Can you work these out from the drawing? Everything is in mm from the part's minimum corner. Coordinates: 2 decimals unless noted, no trailing zeros. Write each loop counter-clockwise with the first axis right and the second up, starting at its lowest first coordinate (ties: lowest second). Pieces come first, ordered by that corner, then holes.
(1) Thinking about a two-plate mould opening in Y: for the marked faces 1, 2 and 3, which applies, released by +Y, released by -Y, zero draft, split by the parting line, or undercut?
(2) Imagine slicing it at A-A, the plane x = 22.5. List the corners of the cut face in (y, z) for me.
(3) Imagine slicing it at B-B, the plane y = 22.5. List the corners of the cut face in (x, z) for me, plus the area to 3 significant figures.
(4) Imagine slicing it at D-D, the plane x = 30.5. List the corners of the cut face in (y, z) for me, plus the area to 3 significant figures.
(5) Imagine slicing it at C-C, the plane z = 124. List the corners of the cut face in (x, y) for me, plus the area to 3 significant figures.
(6) Please list where these lines run through material, in increasing order: probe 1 along X at (y, z) = (22, 92); probe 2 along Z at (x, y) = (20, 41); probe 3 along Y at (x, z) = (12.5, 86).
(7) For pin 1 Ø20 at (x, y) = (22.5, 22.5) entering from -Z; pin 2 Ø8 at (y, z) = (11, 28.5) entering from +X; pin 3 Ø3 at (x, z) = (22, 20.5) entering from +Y; pin 4 Ø1.8 at (x, y) = (24.5, 42) entering from -Z, each with a flat end and sliding along its axis, tell me the tip position at first contact or that it passes through.
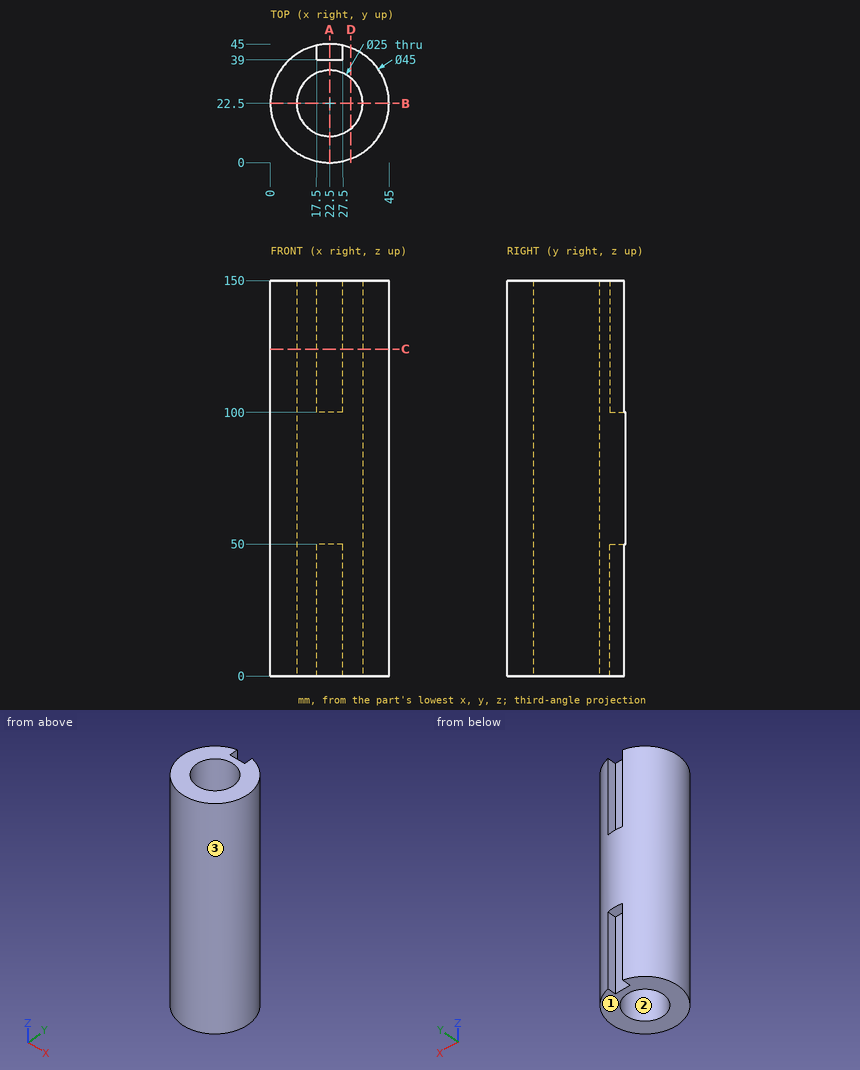
Recorded:
1. face 1: zero draft
1. face 2: undercut
1. face 3: split by the parting line
2. outline: (0, 0) - (10, 0) - (10, 150) - (0, 150) - close; (35, 0) - (39, 0) - (39, 50) - (45, 50) - (45, 100) - (39, 100) - (39, 150) - (35, 150) - close
3. outline: (0, 0) - (10, 0) - (10, 150) - (0, 150) - close; (35, 0) - (45, 0) - (45, 150) - (35, 150) - close
3. area: 3,000 mm2
4. outline: (1.47, 0) - (12.9, 0) - (12.9, 150) - (1.47, 150) - close; (32.1, 0) - (43.53, 0) - (43.53, 150) - (32.1, 150) - close
4. area: 3,430 mm2
5. outline: (17.5, 39) - (17.5, 44.44) arc R22.5 ccw (long way) to (27.5, 44.44) - (27.5, 39) - close; hole circle Ø25 at (22.5, 22.5)
5. area: 1,040 mm2
6. probe 1: x = 0.01 to 10.01, 34.99 to 44.99
6. probe 2: z = 50 to 100
6. probe 3: y = 2.34 to 15, 30 to 42.66
7. pin 1: passes through
7. pin 2: stops at x = 43.71
7. pin 3: stops at y = 39
7. pin 4: stops at z = 50
